Geometry check sheet. Reference: the model listing, model coordinates, mm. Round coordinates to 2 decimals unless told otherwise and drop trailing zeros. Loops run counter-clockwise (first coordinate to the right, second up) from the corner with the lowest first, then second, coordinate; pieces in that order, holes last. Notation, with made-up numbers: M 13.25,68.5 L 27.25,68.5 A19 ccw 27.25,75.5 Z; hole C 25,-25.75 d2. An arc over 180 degrees is marked long. Answer in a Markdown table with one row per item. Add a question column.
```python
from build123d import *

# Parameters (mm, degrees)
SKETCH1_W           = 160
SKETCH1_H           = 60
BOSS_EXTRUDE1_DEPTH = 3
SKETCH2_W           = 51.046896962
SKETCH2_H           = 33.928778657
CUT_EXTRUDE1_DEPTH  = 171.906407136
FILLET1_R           = 2


with BuildPart() as part:
    # Sketch1 → Boss-Extrude1 (new body)
    with BuildSketch(Plane.XY):
        with Locations((80, 30)):
            Rectangle(SKETCH1_W, SKETCH1_H)
    extrude(amount=BOSS_EXTRUDE1_DEPTH)

    # Sketch2 → Cut-Extrude1 (cut, through all)
    with BuildSketch(Plane(origin=(0, 0, 0), x_dir=(-1, 0, 0), z_dir=(0, 0, -1))):
        with Locations((-80, 34.206093002)):
            Rectangle(SKETCH2_W, SKETCH2_H)
    extrude(amount=-CUT_EXTRUDE1_DEPTH, mode=Mode.SUBTRACT)

    # Fillet1
    fillet1_edges = [part.edges().sort_by_distance(p)[0] for p in [
        (160, 30, 0),
        (80, 0, 0),
        (0, 30, 0),
    ]]
    fillet(fillet1_edges, radius=FILLET1_R)


solid = part.part
```
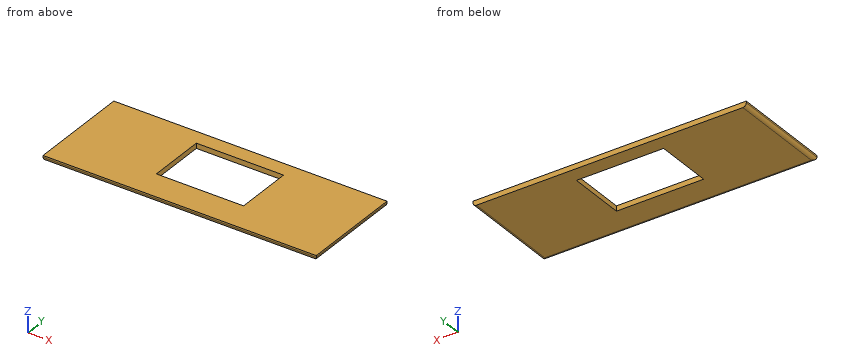
1) Cross-section at C-C, the plane y = 44. Record the boundary of the cut face in (x, z), plus the area to 3 significant figures.
2) Cross-section at A-A, the plane z = 2.5. Record the boundary of the cut face in (x, y).
3) Cross-section at B-B, the plane x = 88. Record the boundary of the cut face in (y, z), plus the area to 3 significant figures.
4) Thickness scan on L1, parallel to X at y = 45.5, z = 2.6; L2, parallel to Y at x = 56, z = 0.85; L3, parallel to Y at x = 87, z = 0.6. Record the ranges inside material, lowest first. Write a range as [from, to].
Worked answers:
| question | item | result |
|---|---|---|
| 1 | outline | M 0,2 A2 ccw 2,0 L 54.48,0 L 54.48,3 L 0,3 Z; M 105.52,0 L 158,0 A2 ccw 160,2 L 160,3 L 105.52,3 Z |
| 1 | area | 325 mm2 |
| 2 | outline | M 0,0 L 160,0 L 160,60 L 0,60 Z; hole M 54.48,17.24 L 105.52,17.24 L 105.52,51.17 L 54.48,51.17 Z |
| 3 | outline | M 0,2 A2 ccw 2,0 L 17.24,0 L 17.24,3 L 0,3 Z; M 51.17,0 L 60,0 L 60,3 L 51.17,3 Z |
| 3 | area | 77.4 mm2 |
| 4 | L1 | x = [0, 54.48], [105.52, 160] |
| 4 | L2 | y = [0.36, 17.24], [51.17, 60] |
| 4 | L3 | y = [0.57, 17.24], [51.17, 60] |
